from build123d import *

# Parameters (mm, degrees)
F0_W     = 90
F0_H     = 90
F1_DEPTH = 13
F2_W     = 87.5
F2_H     = 87.5
F3_DEPTH = 12
F4_R     = 3


with BuildPart() as f1:
    # F0 (on Top) → F1 (new body)
    with BuildSketch(Plane.XY):
        Rectangle(F0_W, F0_H)
    extrude(amount=F1_DEPTH)

    # F2 (on face) → F3 (cut)
    with BuildSketch(Plane.XY.offset(13)):
        Rectangle(F2_W, F2_H)
    extrude(amount=-F3_DEPTH, mode=Mode.SUBTRACT)

    # F4
    f4_edges = [f1.edges().sort_by_distance(p)[0] for p in [
        (45, 0, 0),
        (0, 45, 0),
        (-45, 0, 0),
        (0, -45, 0),
        (45, -45, 6.5),
        (45, 45, 6.5),
        (-45, -45, 6.5),
        (-45, 45, 6.5),
        (-43.75, 0, 1),
        (0, -43.75, 1),
        (43.75, 0, 1),
        (0, 43.75, 1),
        (-43.75, 43.75, 7),
        (43.75, 43.75, 7),
        (43.75, -43.75, 7),
        (-43.75, -43.75, 7),
    ]]
    fillet(f4_edges, radius=F4_R)


solid = f1.part
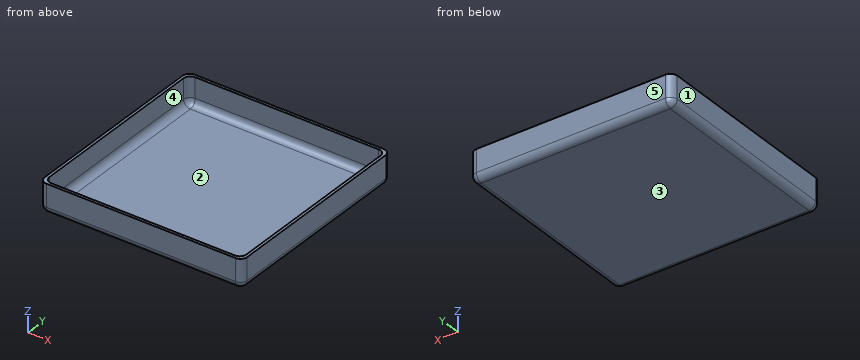
Check sheet for the modelled part. Datum: model origin and axes. Units: mm. Face numbers are marked on the shaded views. A direction names the side the tool comes from. Round coordinates to 2 decimals unless told otherwise and drop trailing zeros. Loops run counter-clockwise (first coordinate to the right, second up) from the corner with the lowest first, then second, coordinate; pieces in that order, holes last.
1. Gauge pin test, flat ends, axial feed: pin 1 Ø4 at (y, z) = (3.5, 2.5) entering from -X; pin 2 Ø1.5 at (x, y) = (-11, 18.5) entering from +Z. Record the tip position at first contact, or that the pin passes through.
2. Sectioned sample at B-B on y = 1.5. Record the boundary of the cut face in (x, z).
3. Sectioned sample at A-A on z = 6.25. Record the boundary of the cut face in (x, y), and give its area (3 significant figures).
4. Set-up check for the marked faces 4 and 5: record each of +Z, -Z, +X, -X, +Y, -Y from which the full face is reachable in a straight line by a thin tool's end or side.
5. Mould release check, pull along X, two halves, no side actions. Record for the marked faces 1, 2 and 3: released by +X, released by -X, zero draft, split by the parting line, or undercut.
6. Scan lines: probe 1 along Y at (x, z) = (-30, 11.75); probe 2 along Z at (x, y) = (10, 2). Record each from-to range of solid material in increasing order.
Recorded:
1. pin 1: stops at x = -45
1. pin 2: stops at z = 1
2. outline: (-45, 3) arc R3 ccw to (-42, 0) - (42, 0) arc R3 ccw to (45, 3) - (45, 13) - (43.75, 13) - (43.75, 4) arc R3 cw to (40.75, 1) - (-40.75, 1) arc R3 cw to (-43.75, 4) - (-43.75, 13) - (-45, 13) - close
3. outline: (-45, -42) arc R3 ccw to (-42, -45) - (42, -45) arc R3 ccw to (45, -42) - (45, 42) arc R3 ccw to (42, 45) - (-42, 45) arc R3 ccw to (-45, 42) - close; hole (-43.75, -40.75) arc R3 ccw to (-40.75, -43.75) - (40.75, -43.75) arc R3 ccw to (43.75, -40.75) - (43.75, 40.75) arc R3 ccw to (40.75, 43.75) - (-40.75, 43.75) arc R3 ccw to (-43.75, 40.75) - close
3. area: 444 mm2
4. face 4: +Z
4. face 5: +Z, -Z, +X, -X, +Y
5. face 1: released by -X
5. face 2: undercut
5. face 3: zero draft
6. probe 1: y = -45 to -43.75, 43.75 to 45
6. probe 2: z = 0 to 1
